from build123d import *

# Parameters (mm, degrees)
SKETCH_1_W                         = 200
SKETCH_1_H                         = 300
SM_BASE_FLANGE_1_DEPTH             = 2
SM_EDGE_FLANGE_1_STRIP_W           = 8.2
SM_EDGE_FLANGE_1_STRIP_H           = 2
SM_EDGE_FLANGE_1_STRIP_CUT_DEPTH   = 300
SM_EDGE_FLANGE_1_STRIP_2_W         = 8.2
SM_EDGE_FLANGE_1_STRIP_2_H         = 2
SM_EDGE_FLANGE_1_STRIP_CUT_2_DEPTH = 300
SM_EDGE_FLANGE_1_DEPTH             = 300
SM_EDGE_FLANGE_1_BEND_DEPTH        = 300


# Sheet-metal steps are written as plain solids
with BuildPart() as part:
    # Sketch 1 → 基体-法兰1 (new body)
    with BuildSketch(Plane.XY):
        Rectangle(SKETCH_1_W, SKETCH_1_H)
    extrude(amount=-SM_BASE_FLANGE_1_DEPTH)

    # 边线-法兰1 strip (across the edge) → 边线-法兰1 strip cut (cut)
    with BuildSketch(Plane(origin=(100, 150, -2), x_dir=(-1, 0, 0), z_dir=(0, -1, 0))):
        with Locations((-2, -1)):
            Rectangle(SM_EDGE_FLANGE_1_STRIP_W, SM_EDGE_FLANGE_1_STRIP_H)
    extrude(amount=SM_EDGE_FLANGE_1_STRIP_CUT_DEPTH, mode=Mode.SUBTRACT)

    # 边线-法兰1 strip 2 (across the edge) → 边线-法兰1 strip cut 2 (cut)
    with BuildSketch(Plane(origin=(-100, -150, -2), x_dir=(1, 0, 0), z_dir=(0, 1, 0))):
        with Locations((-2, -1)):
            Rectangle(SM_EDGE_FLANGE_1_STRIP_2_W, SM_EDGE_FLANGE_1_STRIP_2_H)
    extrude(amount=SM_EDGE_FLANGE_1_STRIP_CUT_2_DEPTH, mode=Mode.SUBTRACT)

    # 边线-法兰1 section (across the edge) → 边线-法兰1 (add)
    with BuildSketch(Plane(origin=(100, 150, -2), x_dir=(-1, 0, 0), z_dir=(0, -1, 0))):
        with BuildLine():
            Line((0, 0.1), (0, 18))
            Line((0, 18), (2, 18))
            Line((2, 18), (2, 0.1))
            ThreePointArc((2, 0.1), (2.029289322, 0.029289322), (2.1, 0))
            Line((2.1, 0), (2.1, -2))
            ThreePointArc((2.1, -2), (0.61507576, -1.38492424), (0, 0.1))
        make_face()
    extrude(amount=SM_EDGE_FLANGE_1_DEPTH)

    # 边线-法兰1 section 2 (across the edge) → 边线-法兰1 bend (add)
    with BuildSketch(Plane(origin=(-100, -150, -2), x_dir=(1, 0, 0), z_dir=(0, 1, 0))):
        with BuildLine():
            Line((0, 0.1), (0, 18))
            Line((0, 18), (2, 18))
            Line((2, 18), (2, 0.1))
            ThreePointArc((2, 0.1), (2.029289322, 0.029289322), (2.1, 0))
            Line((2.1, 0), (2.1, -2))
            ThreePointArc((2.1, -2), (0.61507576, -1.38492424), (0, 0.1))
        make_face()
    extrude(amount=SM_EDGE_FLANGE_1_BEND_DEPTH)


solid = part.part
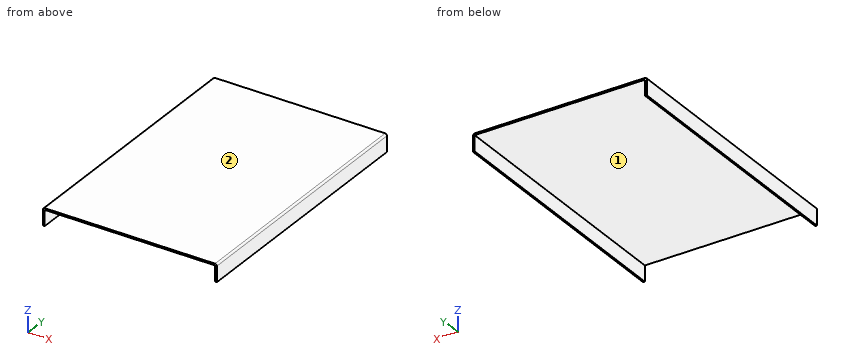
Could you check a few things on this model? Use its own coordinates, in mm. Face numbers are marked on the shaded views. Give positions to 0.01 mm unless a question says otherwise; leave off trailing zeros. Write each loop counter-clockwise with the first axis right and the second up, starting at its lowest first coordinate (ties: lowest second). Pieces come first, ordered by that corner, then holes. Notation, with made-up numbers: (51.25, 15.25) -> (58.25, 15.25) arc R18 cw to (58.25, 37.25) -> close; hole circle Ø10 at (6.5, -3.5). An arc over 180 degrees is marked (long way). Write each question's results on one line, items separated by ' | '. Start each with the question number.
Q1. I'm going to push a flat-ended pin straight in: pin 1 Ø2 at (x, y) = (-48, 101) entering from -Z. Where does the tip first touch, or does it pass through?
Q2. Suppose I cut it at B-B, the plane y = 128.5. List the corners of the cut face in (x, z) for me, and give its area (3 significant figures).
Q3. We'd pull the mould along X, two halves only. Please class the marked faces 1 and 2: +X half, -X half, draft (parallel to the pull), parting line (faces both ways), or undercut.
Q4. I need wall thicknesses on probe 1 along X at (y, z) = (-24.5, -14.25); probe 2 along Z at (x, y) = (-61, -29); probe 3 along X at (y, z) = (-62.5, -1.25). Which ranges of each line are inside material? Lowest first, please.
Q5. Suppose I cut it at A-A, the plane z = -5.25. List the corners of the cut face in (x, y) for me, and give its area (3 significant figures).
Q6. Suppose I cut it at C-C, the plane x = 42. List the corners of the cut face in (y, z) for me, and give its area (3 significant figures).
Outcome:
1) pin 1: z = -2
2) outline: (-100, -20) -> (-98, -20) -> (-98, -2.1) arc R0.1 cw to (-97.9, -2) -> (97.9, -2) arc R0.1 cw to (98, -2.1) -> (98, -20) -> (100, -20) -> (100, -2.1) arc R2.1 ccw to (97.9, 0) -> (-97.9, 0) arc R2.1 ccw to (-100, -2.1) -> close | area: 470 mm2
3) face 1: undercut | face 2: draft
4) probe 1: -100 to -98, 98 to 100 | probe 2: -2 to 0 | probe 3: -99.82 to 99.82
5) outline: (-100, -150) -> (-98, -150) -> (-98, 150) -> (-100, 150) -> close; (98, -150) -> (100, -150) -> (100, 150) -> (98, 150) -> close | area: 1,200 mm2
6) outline: (-150, -2) -> (150, -2) -> (150, 0) -> (-150, 0) -> close | area: 600 mm2
